from build123d import *

# Parameters (mm, degrees)
SKETCH1_R           = 2.1
SKETCH1_R_2         = 3.05
BOSS_EXTRUDE1_DEPTH = 11
FILLET1_R           = 2.5
SKETCH3_W           = 62.051099289
SKETCH3_H           = 53.114404745
CUT_EXTRUDE2_DEPTH  = 1


with BuildPart() as part:
    # Sketch1 → Boss-Extrude1 (new body)
    with BuildSketch(Plane(origin=(0, 0, 0), x_dir=(1, 0, 0), z_dir=(0, 1, 0))):
        with BuildLine():
            Line((-141.618040472, -49.123128832), (-141.618040472, -47.605232566))
            ThreePointArc((-141.618040472, -47.605232566), (-142.400064406, -45.070147956), (-141.618040472, -42.535063347))
            Line((-141.618040472, -42.535063347), (-141.618040472, -12.337528489))
            ThreePointArc((-141.618040472, -12.337528489), (-137.391041816, -7.146645093), (-132.135757115, -2.999987309))
            Line((-132.135757115, -2.999987309), (-104.000008179, -2.999987309))
            ThreePointArc((-104.000008179, -2.999987309), (-100.000008179, -6.999987309), (-104.000008179, -10.999987309))
            Line((-104.000008179, -10.999987309), (-108.800450344, -10.999987309))
            ThreePointArc((-108.800450344, -10.999987309), (-115.958519489, -28.95773414), (-133.507163129, -37.067218191))
            Line((-133.507163129, -37.067218191), (-133.507163129, -41.760704141))
            ThreePointArc((-133.507163129, -41.760704141), (-134.203416554, -49.142591284), (-141.618040472, -49.123128832))
        make_face()
        with Locations(Location((-104.000008179, -6.999987309, 0), (0, 0, 270))):
            Circle(SKETCH1_R, mode=Mode.SUBTRACT)
        with Locations(Location((-120, -7, 0), (0, 0, 270))):
            Circle(SKETCH1_R, mode=Mode.SUBTRACT)
        with Locations(Location((-137.900064406, -45.070147956, 0), (0, 0, 270))):
            Circle(SKETCH1_R_2, mode=Mode.SUBTRACT)
        with BuildLine():
            Line((-115.253720782, -11.000000067), (-131.784308422, -11.000000067))
            ThreePointArc((-131.784308422, -11.000000067), (-133.511366358, -12.688858412), (-135.059388776, -14.543204177))
            Line((-135.059388776, -14.543204177), (-135.07674933, -30.650657269))
            ThreePointArc((-135.07674933, -30.650657269), (-121.070295096, -24.956188563), (-115.253720782, -11.000000067))
        make_face(mode=Mode.SUBTRACT)
    extrude(amount=BOSS_EXTRUDE1_DEPTH)

    # Fillet1
    fillet1_edges = [part.edges().sort_by_distance(p)[0] for p in [
        (-141.618040472, 5.5, 47.605232566),
        (-141.618040472, 5.5, 42.535063347),
        (-132.135757115, 5.5, 2.999987309),
        (-108.800450344, 5.5, 10.999987309),
        (-133.507163129, 5.5, 37.067218191),
        (-135.07674933, 5.5, 30.650657269),
        (-115.253720782, 5.5, 11.000000067),
        (-131.784308422, 5.5, 11.000000067),
        (-135.059388776, 5.5, 14.543204177),
    ]]
    fillet(fillet1_edges, radius=FILLET1_R)

    # Sketch3 → Cut-Extrude2 (cut)
    with BuildSketch(Plane.XZ):
        with Locations((-120.556091454, 37.557189682)):
            Rectangle(SKETCH3_W, SKETCH3_H)
    extrude(amount=-CUT_EXTRUDE2_DEPTH, mode=Mode.SUBTRACT)


solid = part.part
Geometry check sheet. Reference: the model listing, model coordinates, mm. A direction names the side the tool comes from. Give positions to 0.01 mm unless a question says otherwise; leave off trailing zeros. Order: outer loops, then holes, each group sorted by start corner. A loop starts at its lowest first (then second) coordinate and runs counter-clockwise, first axis right, second up. Notation, with made-up numbers: M 17.5,-0.5 L 38.5,-0.5 A9 ccw 38.5,9.5 Z; hole C -39,-15.5 d2. An arc over 180 degrees is marked long. Use a Markdown table: item, result.
Item 1: Section check B-B (z = 7). Record the cut outline in (x, y), and give its area (3 significant figures).
Answers follow:
| item | result |
|---|---|
| outline | M -137.24,0 L -122.1,0 L -122.1,11 L -137.24,11 Z; M -117.9,0 L -106.1,0 L -106.1,11 L -117.9,11 Z; M -101.9,0 L -100,0 L -100,11 L -101.9,11 Z |
| area | 317 mm2 |
Item 2: Tool access check on faces 1 (the cylindrical face through (-132.908, 6.07, 37.714)), 2 (the flat face through (-115.5, 0.6, 11)), 3 (the flat face through (-128, 1, 31)), 4 (the cylindrical face through (-134.2, 6.07, 29.89)), 5 (the flat face through (-141.618, 6, 27)). Record the directions out of +Z, -Z, +X, -X, +Y, -Y that give a thin tool (end or side, any length) a straight path to the whole face; none if there is none.
Answers follow:
| item | result |
|---|---|
| face 1 | +X, +Y, -Y |
| face 2 | +Z, +X, -Y |
| face 3 | +Z, +X, -X, -Y |
| face 4 | +Y, -Y |
| face 5 | -Z, -X, +Y, -Y |
Item 3: Material ranges on line 1 along X through (y, z) = (5.75, 7); line 2 along X through (y, z) = (9.5, 7.5); line 3 along X through (y, z) = (7, 13), recorded low to high.
Answers follow:
| item | result |
|---|---|
| line 1 | x = -137.24 to -122.1, -117.9 to -106.1, -101.9 to -100 |
| line 2 | x = -137.74 to -122.04, -117.96 to -106.04, -101.96 to -100.03 |
| line 3 | x = -141.62 to -133.79, -115.49 to -108.86 |
Item 4: Section check D-D (y = 3). Record the cut outline in (x, z), and give its area (3 significant figures).
Answers follow:
| item | result |
|---|---|
| outline | M -141.9,43 A2.5 cw -141.62,41.86 L -141.62,12.34 A30.58 ccw -132.78,3.41 A2.5 ccw -131.4,3 L -104,3 A4 ccw -104,11 L -106.41,11 A2.5 cw -108.9,13.28 A26.1 ccw -131.35,36.86 A2.5 cw -133.51,39.34 L -133.51,41.76 A5.5 ccw -141.62,49.12 L -141.62,48.29 A2.5 cw -141.9,47.14 A4.5 ccw Z; hole C -137.9,45.07 d6.1; hole M -135.07,27.99 L -135.06,15.4 A2.5 ccw -134.5,13.83 A23.93 ccw -132.54,11.7 A2.5 ccw -130.81,11 L -117.94,11 A2.5 ccw -115.46,13.86 A19.65 ccw -132.23,30.47 A2.5 ccw Z; hole C -120,7 d4.2; hole C -104,7 d4.2 |
| area | 759 mm2 |
Item 5: Section check A-A (x = -120). State how many separate pieces and enclosed holes the cut face has, and give its area (3 significant figures).
Answers follow:
| item | result |
|---|---|
| separate pieces | 3 |
| enclosed holes | 0 |
| area | 128 mm2 |
Item 6: Draft check along X on faces 6 (the flat face through (-120, 0, 10)), 7 (the cylindrical face through (-100, 5, 7)), 8 (the cylindrical face through (-134.92, 6.07, 14.58)). Enter one of: +X half, -X half, draft (parallel to the pull), parting line (faces both ways), or undercut.
Answers follow:
| item | result |
|---|---|
| face 6 | draft |
| face 7 | +X half |
| face 8 | undercut |
Item 7: Depth check by flat-ended pin: P1, Ø2, axis at y = 1.5, z = 32, coming from the +X side; P2, Ø10, axis at x = -137.9, z = 45.07, coming from the +Y side; P3, Ø3, axis at x = -114, z = 31.5, coming from the -Y side; P4, Ø2, axis at x = -134.5, y = 9, coming from the +Z side. Enter the tip coordinate at first touch or a pass-through.
Answers follow:
| item | result |
|---|---|
| P1 | stops at x = -118.13 |
| P2 | stops at y = 11 |
| P3 | passes through |
| P4 | stops at z = 50.02 |
Item 8: Section check C-C (z = 20.5). Record the cut outline in (x, y), and give its area (3 significant figures).
Answers follow:
| item | result |
|---|---|
| outline | M -141.62,1 L -135.07,1 L -135.07,11 L -141.62,11 Z; M -117.7,1 L -110.59,1 L -110.59,11 L -117.7,11 Z |
| area | 137 mm2 |
